Can you work these out from the model? Positions are in its coordinate system, mm. A direction names the side the tool comes from. Round coordinates to 2 decimals unless told otherwise and drop trailing zeros. Write each loop counter-clockwise with the first axis right and the second up, starting at its lowest first coordinate (ties: lowest second). Pieces come first, ordered by that corner, then holes. Notation, with made-up numbers: (52.5, 85) - (61.5, 85) arc R19 ccw to (61.5, 97) - close; hole circle Ø5 at (15.25, 10.25). An arc over 180 degrees is marked (long way). One line per item, written item: value. Start each with the question number.
(1) On a 3-axis mill with a long thin cutter (end or side, diameter ignored), from which of +Z, -Z, +X, -X, +Y, -Y can I reach the whole of each face in a straight line? I mean faces 1 (the face through (-25, -16, -25.4)), 2 (the face through (-8.948, -40.293, 11.27)), 3 (the face through (35, -11, -2.54)), 4 (the face through (13.559, 46.845, -34.881)), 5 (the face through (-46.79, -4.34, -24.15)). Say none if no direction works.
(2) I want a section at C-C on z = 8. List the corners of the cut face in (x, y) for me (3 decimals).
(3) If I drill on L1, parallel to Z at x = 45, y = -23.5; L2, parallel to Y at x = -25, z = -23.5; L3, parallel to Y at x = 0, z = 11.5 (3 decimals), over which ranges is the centre line in solid material (lowest first)? Write a range as from..to.
(4) I want a section at A-A on z = -19.5. List the corners of the cut face in (x, y) for me.
(5) Thinking about a two-plate mould opening in Y: for faces 6 (the face through (0, 43, -20)), 7 (the face through (13, 45, -31.75)), 8 (the face through (-13.001, -47.003, -34.881)), 9 (the face through (-36, 4, -2.54)), which applies, +Y half, -Y half, draft (parallel to the pull), parting line (faces both ways), or undercut?
(6) I'm going to push flat-ended pins straight in: pin 1 Ø10 at (y, z) = (-44.5, -3) entering from -X; pin 2 Ø21.5 at (x, y) = (7, 8) entering from -Z; pin 3 Ø5.5 at (x, y) = (8, 44.5) entering from +Z; pin 4 Ø6 at (y, z) = (-17, 17.5) entering from +X. Where does each tip first touch, or does it pass through?
(7) I want a section at B-B on z = -9.5. List the corners of the cut face in (x, y) for me, plus the area to 3 significant figures.
from build123d import *

# Parameters (mm, degrees)
SKETCH1_R           = 41.275
BOSS_EXTRUDE1_DEPTH = 25.4
SKETCH2_R           = 36.068
CUT_EXTRUDE1_DEPTH  = 25.4
SKETCH3_R           = 57.15
BOSS_EXTRUDE2_DEPTH = 25.4
SKETCH4_R           = 29.21
CUT_EXTRUDE2_DEPTH  = 96.461432003
CUT_EXTRUDE4_DEPTH  = 22.86
CUT_EXTRUDE5_DEPTH  = 20.32
BOSS_EXTRUDE3_DEPTH = 6.35
BOSS_EXTRUDE4_DEPTH = 6.35
BOSS_EXTRUDE5_DEPTH = 6.35
BOSS_EXTRUDE6_DEPTH = 6.35
CUT_EXTRUDE6_DEPTH  = 22.86
CUT_EXTRUDE7_DEPTH  = 20.32
SKETCH15_R          = 34.29
SKETCH15_R_2        = 30.48
CUT_EXTRUDE8_DEPTH  = 12.7
FILLET1_R           = 2.54


with BuildPart() as part:
    # Sketch1 → Boss-Extrude1 (new body)
    with BuildSketch(Plane.XY):
        Circle(SKETCH1_R)
    extrude(amount=BOSS_EXTRUDE1_DEPTH)

    # Sketch2 → Cut-Extrude1 (cut)
    with BuildSketch(Plane.XY.offset(25.4)):
        Circle(SKETCH2_R)
    extrude(amount=-CUT_EXTRUDE1_DEPTH, mode=Mode.SUBTRACT)

    # Sketch3 → Boss-Extrude2 (add)
    with BuildSketch(Plane(origin=(0, 0, 0), x_dir=(-1, 0, 0), z_dir=(0, 0, -1))):
        Circle(SKETCH3_R)
    extrude(amount=BOSS_EXTRUDE2_DEPTH)

    # Sketch4 → Cut-Extrude2 (cut, through all)
    with BuildSketch(Plane(origin=(0, 0, -25.4), x_dir=(-1, 0, 0), z_dir=(0, 0, -1))):
        Circle(SKETCH4_R)
    extrude(amount=-CUT_EXTRUDE2_DEPTH, mode=Mode.SUBTRACT)

    # Sketch6 → Cut-Extrude4 (cut)
    with BuildSketch(Plane(origin=(0, 0, -25.4), x_dir=(-1, 0, 0), z_dir=(0, 0, -1))):
        with BuildLine():
            Line((18.506279238, -30.364967129), (24.454726136, -40.125135135))
            ThreePointArc((24.454726136, -40.125135135), (46.842589674, -3.719125253), (30.48, 35.763524714))
            ThreePointArc((30.48, 35.763524714), (28.349648711, 38.283083694), (27.139008157, 41.35243599))
            ThreePointArc((27.139008157, 41.35243599), (26.51640571, 42.835799248), (25.4, 43.994090512))
            ThreePointArc((25.4, 43.994090512), (13.148007491, 49.069031975), (0, 50.8))
            Line((0, 50.8), (0, 35.56))
            ThreePointArc((0, 35.56), (34.23661659, 9.610810811), (18.506279238, -30.364967129))
        make_face()
    extrude(amount=-CUT_EXTRUDE4_DEPTH, mode=Mode.SUBTRACT)

    # Sketch8 → Cut-Extrude5 (cut)
    with BuildSketch(Plane(origin=(0, 0, -22.86), x_dir=(-1, 0, 0), z_dir=(0, 0, -1))):
        with BuildLine():
            Line((26.437541769, -43.37852447), (24.454726136, -40.125135135))
            ThreePointArc((24.454726136, -40.125135135), (46.842589674, -3.719125253), (30.48, 35.763524714))
            ThreePointArc((30.48, 35.763524714), (28.349648711, 38.283083694), (27.139008157, 41.35243599))
            ThreePointArc((27.139008157, 41.35243599), (26.51640571, 42.835799248), (25.4, 43.994090512))
            ThreePointArc((25.4, 43.994090512), (50.796418637, 0.6032028), (26.437541769, -43.37852447))
        make_face()
    extrude(amount=-CUT_EXTRUDE5_DEPTH, mode=Mode.SUBTRACT)

    # Sketch9 → Boss-Extrude3 (add)
    with BuildSketch(Plane(origin=(0, 0, -25.4), x_dir=(-1, 0, 0), z_dir=(0, 0, -1))):
        with BuildLine():
            Line((0, 44.45), (0, 38.608))
            ThreePointArc((0, 38.608), (-10.589622857, 37.127315439), (-20.36698447, 32.798835461))
            Line((-20.36698447, 32.798835461), (-23.448830804, 37.761817143))
            ThreePointArc((-23.448830804, 37.761817143), (-12.192, 42.745264486), (0, 44.45))
        make_face()
    extrude(amount=BOSS_EXTRUDE3_DEPTH)

    # Sketch10 → Boss-Extrude4 (add)
    with BuildSketch(Plane(origin=(0, 0, -31.75), x_dir=(-1, 0, 0), z_dir=(0, 0, -1))):
        with BuildLine():
            Line((-20.36698447, 32.798835461), (-25.726717225, 41.430107951))
            ThreePointArc((-25.726717225, 41.430107951), (-13.376365714, 46.897661608), (0, 48.768))
            Line((0, 48.768), (0, 38.608))
            ThreePointArc((0, 38.608), (-10.589622857, 37.127315439), (-20.36698447, 32.798835461))
        make_face()
    extrude(amount=BOSS_EXTRUDE4_DEPTH)

    # Sketch11 → Boss-Extrude5 (add)
    with BuildSketch(Plane(origin=(0, 0, -25.4), x_dir=(-1, 0, 0), z_dir=(0, 0, -1))):
        with BuildLine():
            Line((0, -46.228), (0, -38.608))
            ThreePointArc((0, -38.608), (10.434594595, -37.171183727), (20.092531744, -32.967678598))
            Line((20.092531744, -32.967678598), (24.058163009, -39.474457268))
            ThreePointArc((24.058163009, -39.474457268), (12.494054054, -44.507601568), (0, -46.228))
        make_face()
    extrude(amount=BOSS_EXTRUDE5_DEPTH)

    # Sketch12 → Boss-Extrude6 (add)
    with BuildSketch(Plane(origin=(0, 0, -31.75), x_dir=(-1, 0, 0), z_dir=(0, 0, -1))):
        with BuildLine():
            Line((0, -38.608), (0, -48.768))
            ThreePointArc((0, -48.768), (13.180540541, -46.953074181), (25.380040098, -41.643383492))
            Line((25.380040098, -41.643383492), (20.092531744, -32.967678598))
            ThreePointArc((20.092531744, -32.967678598), (10.434594595, -37.171183727), (0, -38.608))
        make_face()
    extrude(amount=BOSS_EXTRUDE6_DEPTH)

    # Sketch13 → Cut-Extrude6 (cut)
    with BuildSketch(Plane(origin=(0, 0, -25.4), x_dir=(-1, 0, 0), z_dir=(0, 0, -1))):
        with BuildLine():
            Line((0, -35.56), (0, -50.8))
            ThreePointArc((0, -50.8), (-13.148007491, -49.069031975), (-25.4, -43.994090512))
            ThreePointArc((-25.4, -43.994090512), (-27.380071612, -41.913162133), (-27.914964156, -39.090957945))
            ThreePointArc((-27.914964156, -39.090957945), (-29.023609665, -37.293207394), (-30.48, -35.763524714))
            ThreePointArc((-30.48, -35.763524714), (-46.857702082, 3.52361399), (-24.788763993, 39.919635265))
            Line((-24.788763993, 39.919635265), (-18.759064643, 30.209453714))
            ThreePointArc((-18.759064643, 30.209453714), (-34.196211589, -9.7536), (0, -35.56))
        make_face()
    extrude(amount=-CUT_EXTRUDE6_DEPTH, mode=Mode.SUBTRACT)

    # Sketch14 → Cut-Extrude7 (cut)
    with BuildSketch(Plane(origin=(0, 0, -22.86), x_dir=(-1, 0, 0), z_dir=(0, 0, -1))):
        with BuildLine():
            Line((-26.798663776, 43.156362449), (-24.788763993, 39.919635265))
            ThreePointArc((-24.788763993, 39.919635265), (-46.857702082, 3.52361399), (-30.48, -35.763524714))
            ThreePointArc((-30.48, -35.763524714), (-29.023609665, -37.293207394), (-27.914964156, -39.090957945))
            ThreePointArc((-27.914964156, -39.090957945), (-27.380071612, -41.913162133), (-25.4, -43.994090512))
            ThreePointArc((-25.4, -43.994090512), (-50.793459105, -0.815176157), (-26.798663776, 43.156362449))
        make_face()
    extrude(amount=-CUT_EXTRUDE7_DEPTH, mode=Mode.SUBTRACT)

    # Sketch15 → Cut-Extrude8 (cut)
    with BuildSketch(Plane(origin=(0, 0, -25.4), x_dir=(-1, 0, 0), z_dir=(0, 0, -1))):
        Circle(SKETCH15_R)
        Circle(SKETCH15_R_2, mode=Mode.SUBTRACT)
    extrude(amount=-CUT_EXTRUDE8_DEPTH, mode=Mode.SUBTRACT)

    # Fillet1
    fillet1_edges = [part.edges().sort_by_distance(p)[0] for p in [
        (57.15, 0, 0),
        (57.15, 0, -25.4),
        (-41.275, 0, 25.4),
    ]]
    fillet(fillet1_edges, radius=FILLET1_R)


solid = part.part
Established:
1. face 1: -Z, +X, -X
1. face 2: +Z
1. face 3: none
1. face 4: -Z, +X, +Y
1. face 5: -Z
2. outline: circle Ø82.55 at (0, 0); hole circle Ø72.136 at (0, 0)
3. L1: -25.4..-22.86, -2.54..0
3. L2: -51.3..-39.79, -25.29..-23.47, -17.44..-15.11, 15.11..17.44, 23.47..25.29, 44.22..51.3
3. L3: -41.275..-36.068, 36.068..41.275
4. outline: circle Ø114.3 at (0, 0); circle Ø60.96 at (0, 0); hole circle Ø68.58 at (0, 0); hole circle Ø58.42 at (0, 0); hole (-26.44, -43.38) - (-18.51, -30.36) arc R35.56 cw to (0, 35.56) - (0, 50.8) arc R50.8 ccw to start; hole (0, -50.8) arc R50.8 ccw to (26.8, 43.16) - (18.76, 30.21) arc R35.56 cw to (0, -35.56) - close
5. face 6: undercut
5. face 7: draft
5. face 8: -Y half
5. face 9: undercut
6. pin 1: x = -41.3
6. pin 2: through
6. pin 3: z = 0
6. pin 4: x = 38.83
7. outline: circle Ø114.3 at (0, 0); hole circle Ø58.42 at (0, 0); hole (-26.44, -43.38) - (-18.51, -30.36) arc R35.56 cw to (0, 35.56) - (0, 50.8) arc R50.8 ccw to start; hole (0, -50.8) arc R50.8 ccw to (26.8, 43.16) - (18.76, 30.21) arc R35.56 cw to (0, -35.56) - close
7. area: 4,170 mm2
